```python
from build123d import *

# Parameters (mm, degrees)
SKETCH1_W           = 55
SKETCH1_H           = 55
SKETCH1_W_2         = 11.8
SKETCH1_H_2         = 11.8
BOSS_EXTRUDE1_DEPTH = 8
SKETCH2_W           = 55
SKETCH2_H           = 55
BOSS_EXTRUDE7_DEPTH = 12
SKETCH2_5_W         = 23.6
SKETCH2_5_H         = 7
SKETCH2_5_W_2       = 47
BOSS_EXTRUDE8_DEPTH = 8
SKETCH6_R           = 3.15
CUT_EXTRUDE1_DEPTH  = 44.732139211


with BuildPart() as part:
    # Sketch1 → Boss-Extrude1 (new body)
    with BuildSketch(Plane(origin=(0, 0, 0), x_dir=(1, 0, 0), z_dir=(0, 1, 0))):
        Rectangle(SKETCH1_W, SKETCH1_H)
        with Locations((0, 17.6)):
            Rectangle(SKETCH1_W_2, SKETCH1_H_2, mode=Mode.SUBTRACT)
        with Locations((17.6, 0)):
            Rectangle(SKETCH1_W_2, SKETCH1_H_2, mode=Mode.SUBTRACT)
        with Locations((-17.6, 0)):
            Rectangle(SKETCH1_W_2, SKETCH1_H_2, mode=Mode.SUBTRACT)
        with Locations((0, -17.6)):
            Rectangle(SKETCH1_W_2, SKETCH1_H_2, mode=Mode.SUBTRACT)
    extrude(amount=BOSS_EXTRUDE1_DEPTH)

    # Sketch2 → Boss-Extrude7 (add)
    with BuildSketch(Plane.XZ):
        Rectangle(SKETCH2_W, SKETCH2_H)
        Polygon((-23.5, 23.5), (-5.9, 23.5), (5.9, 23.5), (23.5, 23.5), (23.5, 5.9), (23.5, 3.5), (23.5, -3.5), (23.5, -5.9), (23.5, -23.5), (5.9, -23.5), (-5.9, -23.5), (-23.5, -23.5), (-23.5, -5.9), (-23.5, -3.5), (-23.5, 3.5), (-23.5, 5.9), align=None, mode=Mode.SUBTRACT)
    extrude(amount=BOSS_EXTRUDE7_DEPTH)

    # Sketch2_5 → Boss-Extrude8 (add)
    with BuildSketch(Plane.XZ):
        with Locations((0, 17.6)):
            Rectangle(SKETCH2_5_W, SKETCH2_5_H)
        Rectangle(SKETCH2_5_W_2, SKETCH2_5_H)
        with Locations((0, -17.6)):
            Rectangle(SKETCH2_5_W, SKETCH2_5_H)
    extrude(amount=BOSS_EXTRUDE8_DEPTH)

    # Sketch6 → Cut-Extrude1 (cut, through all)
    with BuildSketch(Plane.XZ.offset(12)):
        with Locations(Location((-23.5, 23.5, 0), (0, 0, 270))):
            Circle(SKETCH6_R)
        with Locations(Location((23.5, 23.5, 0), (0, 0, 270))):
            Circle(SKETCH6_R)
        with Locations(Location((-23.5, -23.5, 0), (0, 0, 270))):
            Circle(SKETCH6_R)
        with Locations(Location((23.5, -23.5, 0), (0, 0, 270))):
            Circle(SKETCH6_R)
    extrude(amount=-CUT_EXTRUDE1_DEPTH, mode=Mode.SUBTRACT)


solid = part.part
```
Check sheet for the modelled part. Datum: model origin and axes. Units: mm. A direction names the side the tool comes from. Give positions to 0.01 mm unless a question says otherwise; leave off trailing zeros. Order: outer loops, then holes, each group sorted by start corner. A loop starts at its lowest first (then second) coordinate and runs counter-clockwise, first axis right, second up. Notation, with made-up numbers: M -27.5,80.5 L -16.5,80.5 A26 ccw -16.5,116.5 Z; hole C -17,47 d6. An arc over 180 degrees is marked long. Answer in a Markdown table with one row per item.
1) Release check for a two-part mould opening along Z. For faces 1 (the flat face through (0, -4, 23.5)), 2 (the flat face through (-25, -12, 0)) record: +Z half, -Z half, draft (parallel to the pull), parting line (faces both ways), or undercut.
Filled sheet:
| item | result |
|---|---|
| face 1 | undercut |
| face 2 | draft |
2) Thickness scan on L1, parallel to X at y = 4.75, z = 2; L2, parallel to Z at x = 12, y = -1.75. Record the ranges inside material, lowest first. Write a range as [from, to].
Filled sheet:
| item | result |
|---|---|
| L1 | x = [-27.5, -23.5], [-11.7, 11.7], [23.5, 27.5] |
| L2 | z = [-27.5, -23.5], [-3.5, 3.5], [23.5, 27.5] |
3) Gauge pin test, flat end, axial feed: P1, Ø8, axis at x = -14, z = -1, coming from the -Y side. Record the tip position at first contact, or that the pin passes through.
Filled sheet:
| item | result |
|---|---|
| P1 | stops at y = -8 |
4) Cross-section at C-C, the plane z = -7.5. Enter the section's corners in (x, y).
Filled sheet:
| item | result |
|---|---|
| outline | M -27.5,-12 L -23.5,-12 L -23.5,0 L 23.5,0 L 23.5,-12 L 27.5,-12 L 27.5,8 L -27.5,8 Z |
5) Cross-section at D-D, the plane x = 12.5. Enter the section's corners in (y, z), plus the area to 3 significant figures.
Filled sheet:
| item | result |
|---|---|
| outline | M -12,-27.5 L 8,-27.5 L 8,-5.9 L 0,-5.9 L 0,-23.5 L -12,-23.5 Z; M -12,23.5 L 0,23.5 L 0,5.9 L 8,5.9 L 8,27.5 L -12,27.5 Z; M -8,-3.5 L 0,-3.5 L 0,3.5 L -8,3.5 Z |
| area | 498 mm2 |
6) Cross-section at A-A, the plane y = -4.5. Enter the section's corners in (x, z), plus the area to 3 significant figures.
Filled sheet:
| item | result |
|---|---|
| outline | M -27.5,-27.5 L 27.5,-27.5 L 27.5,27.5 L -27.5,27.5 Z; M -11.8,-21.1 L 11.8,-21.1 L 11.8,-14.1 L -11.8,-14.1 Z; M -11.8,14.1 L 11.8,14.1 L 11.8,21.1 L -11.8,21.1 Z; hole M -23.5,-20.35 A3.15 ccw long -20.35,-23.5 L 20.35,-23.5 A3.15 ccw long 23.5,-20.35 L 23.5,-3.5 L -23.5,-3.5 Z; hole M -23.5,3.5 L 23.5,3.5 L 23.5,20.35 A3.15 ccw long 20.35,23.5 L -20.35,23.5 A3.15 ccw long -23.5,20.35 Z |
| area | 1,380 mm2 |
7) Cross-section at B-B, the plane x = -1.5. Enter the section's corners in (y, z).
Filled sheet:
| item | result |
|---|---|
| outline | M -12,-27.5 L 8,-27.5 L 8,-23.5 L -12,-23.5 Z; M -12,23.5 L 8,23.5 L 8,27.5 L -12,27.5 Z; M -8,-21.1 L 0,-21.1 L 0,-14.1 L -8,-14.1 Z; M -8,-3.5 L 0,-3.5 L 0,-11.7 L 8,-11.7 L 8,11.7 L 0,11.7 L 0,3.5 L -8,3.5 Z; M -8,14.1 L 0,14.1 L 0,21.1 L -8,21.1 Z |
8) Access from +Z, -Z, +X, -X, +Y, -Y to the whole of each face (thin tool, end or side, straight path). Record for faces 3 (the flat face through (0, 4, 11.7)), 4 (the flat face through (0, -8, 0)), 5 (the flat face through (5.9, 4, 18)).
Filled sheet:
| item | result |
|---|---|
| face 3 | +Y, -Y |
| face 4 | -Y |
| face 5 | +Y |
